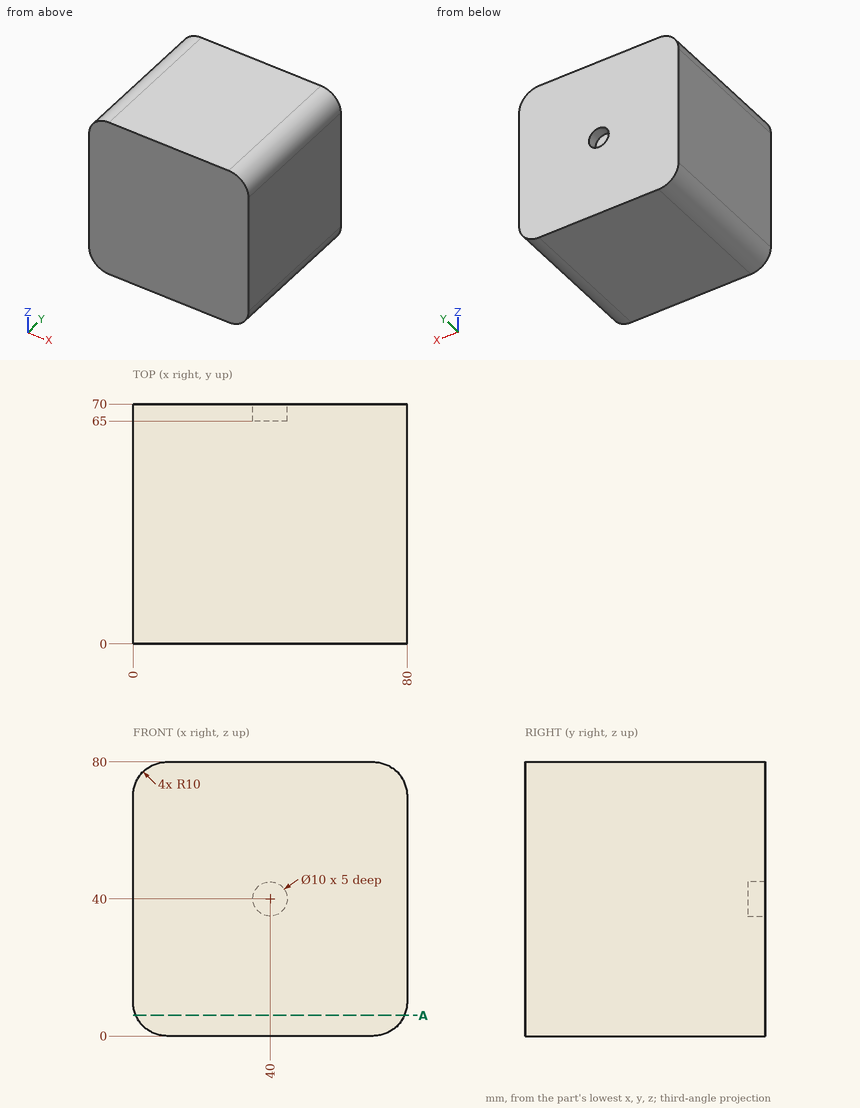
Verification items for this drawing (mm, ordinates from the low corner). Round coordinates to 2 decimals unless told otherwise and drop trailing zeros. Order: outer loops, then holes, each group sorted by start corner. A loop starts at its lowest first (then second) coordinate and runs counter-clockwise, first axis right, second up. Notation, with made-up numbers: (14, 42.5) -> (52, 42.5) arc R19 cw to (52, 63.5) -> close; hole circle Ø3 at (17, -20). An arc over 180 degrees is marked (long way). Use one line per item in the form item = value.
1. Scan lines: line 1 along X through (y, z) = (68.2, 40); line 2 along Y through (x, z) = (44.5, 41); line 3 along Z through (x, y) = (74, 8). Record each from-to range of solid material in increasing order. Write a range as from..to.
Working result:
line_1 = 0..35, 45..80
line_2 = 0..65
line_3 = 0.83..79.17
2. Cross-section at A-A, the plane z = 6. Enter the section's corners in (x, y), plus the area to 3 significant figures.
Working result:
outline = (0.83, 0) -> (79.17, 0) -> (79.17, 70) -> (0.83, 70) -> close
area = 5,480 mm^2
3. Go/stop test with a flat-tipped pin: pin 1 (8 mm diameter, centred on x = 41, z = 40.5, fed in from +Y). Record where the tip stops, or that it passes through.
Working result:
pin_1 = 70
